The model under review builds one solid part; all positions refer to its coordinate system, in mm. A direction names the side the tool comes from. Coordinates: 2 decimals unless noted, no trailing zeros. Write each loop counter-clockwise with the first axis right and the second up, starting at its lowest first coordinate (ties: lowest second). Pieces come first, ordered by that corner, then holes. Notation, with made-up numbers: (87, 33) - (130, 33) arc R21 ccw to (130, 68) - close; hole circle Ø1 at (7.5, 73). An arc over 180 degrees is marked (long way). Answer as CSV lines item,"result". Start each with the question number.
Autodesk Inventor part; units mm, degrees
ref_plane "Work Plane1" through (13.2461, 0.9906, -45.4152) normal (1, 0, 0) x (0, 0, -1)
ref_plane "YZ Plane" through (0, 0, 0) normal (1, 0, 0) x (0, 1, 0)
ref_plane "XZ Plane" through (0, 0, 0) normal (0, 1, 0) x (-1, 0, 0)
sketch "Sketch1" plane through (0, 0, 0) normal (0, 0, 1) x (1, 0, 0)
  line L0 (0, 0) -> (26.4922, 0)
  line L1 (26.4922, 0) -> (26.4922, 17.5006)
  line L2 (26.4922, 17.5006) -> (0, 17.5006)
  line L3 (0, 17.5006) -> (0, 0)
  dimension "d0" = 26.4922
  dimension "d1" = 17.5006
extrude "Extrusion1" add sketch "Sketch1" against normal blind 46.4058
fillet "Fillet1" radius 0.9906 12 edges at (0, 17.5006, -23.2029) (0, 0, -23.2029) (0, 8.7503, 0) (0, 8.7503, -46.4058) (26.4922, 17.5006, -23.2029) (13.2461, 17.5006, 0) (13.2461, 17.5006, -46.4058) (26.4922, 0, -23.2029) (26.4922, 8.7503, 0) (26.4922, 8.7503, -46.4058) (13.2461, 0, 0) (13.2461, 0, -46.4058)
sketch "Sketch2" plane through (0, 0, 0) normal (0, 0, 1) x (1, 0, 0)
  line L0 (0.9906, 16.51) -> (25.5016, 16.51)
  line L1 (0.9906, 0.9906) -> (0.9906, 16.51)
  line L2 (0.9961, 16.5003) -> (25.4961, 16.5003)
  line L3 (0.9961, 16.5003) -> (0.9961, 1.0003)
  line L4 (0.9961, 1.0003) -> (25.4961, 1.0003)
  line L5 (25.4961, 1.0003) -> (25.4961, 16.5003)
  circle A0 centre (6.9961, 8.7503) radius 4.3
  circle A1 centre (19.4961, 8.7503) radius 2.95
  point P0 (0, 0)
  point P1 (13.2461, 8.7503)
  point P2 (13.2461, 8.7503)
  point P3 (13.2461, 16.51)
  point P4 (0.9906, 8.7503)
extrude "Extrusion2" add sketch "Sketch2" along normal blind 3.6068 contours A0 | A1
fillet "Fillet2" radius 0.254 2 edges at (2.6961, 8.7503, 3.6068) (16.5461, 8.7503, 3.6068)
ref_plane "Work Plane1" through (13.2461, 0.9906, -45.4152) normal (1, 0, 0) x (0, 0, -1)
properties part number "276-2243" material "ABS Plastic"
(1) For pin 1 (1 mm diameter, centred on x = 12.5, y = 5.5, fed in from +Z), flat-tipped, find the tip position at first contact; note if it passes through.
(2) For faces 4 (the cylindrical face through (22.22, 9.88, 1.65)), 5 (the cylindrical face through (13.42, 0.3, -0.28)), list the 3-axis set-ups (+Z, -Z, +X, -X, +Y, -Y) from which the entire face can be reached by the end or side of a thin tool; tool diameter is ignored.
(3) Add section B-B on x = 16. Give the boundary of the cut face in (y, z), then the cut area to 3 significant figures.
(4) Wall thickness on line 1 (Z direction, x = 20.5, y = 4.5); line 2 (Z direction, x = 12, y = 0.5): over which ranges is each line inside the solid? List them lowest first.
(5) Add section A-A on y = 2.75. Give the boundary of the cut face in (x, z), then the cut area to 3 significant figures.
(6) The part is to be moulded in two halves that separate along X. For faces 1 (the cylindrical face through (26.19, 8.86, -0.28)), 2 (the cylindrical face through (10.968, 10.397, 1.653)), 3 (the cylindrical face through (0.3, 0.28, -23.51)), say which applies: released by +X, released by -X, zero draft, split by the parting line, or undercut.
Reported:
1,pin 1,"z = 0"
2,face 4,"+Z"
2,face 5,"+Z, +X, -X, -Y"
3,outline,"(0, -45.42) arc R0.99 ccw to (0.99, -46.41) - (16.51, -46.41) arc R0.99 ccw to (17.5, -45.42) - (17.5, -0.99) arc R0.99 ccw to (16.51, 0) - (0.99, 0) arc R0.99 ccw to (0, -0.99) - close"
3,area,"811 mm²"
4,line 1,"-46.41 to 0"
4,line 2,"-46.28 to -0.13"
5,outline,"(0, -45.42) arc R0.99 ccw to (0.99, -46.41) - (25.5, -46.41) arc R0.99 ccw to (26.49, -45.42) - (26.49, -0.99) arc R0.99 ccw to (25.5, 0) - (0.99, 0) arc R0.99 ccw to (0, -0.99) - close"
5,area,"1,230 mm²"
6,face 1,"released by +X"
6,face 2,"undercut"
6,face 3,"released by -X"
